Work out the finished part from the listing and answer in its coordinate system (mm). A direction names the side the tool comes from. Coordinates: 2 decimals unless noted, no trailing zeros. Order: outer loops, then holes, each group sorted by start corner. A loop starts at its lowest first (then second) coordinate and runs counter-clockwise, first axis right, second up. Notation, with made-up numbers: (23.5, 21.25) -> (68.5, 21.25) arc R30 cw to (68.5, 45.25) -> close; hole circle Ø8 at (10.5, -5.5). An arc over 180 degrees is marked (long way). Use one line per item in the form item = value.
from build123d import *

# Parameters (mm, degrees)
F1_DEPTH = 50


with BuildPart() as f1:
    # F0 (on Top) → F1 (new body)
    with BuildSketch(Plane.XY):
        with BuildLine():
            Line((-20.484694, -18.369378), (-21.890144, -14.507935))
            ThreePointArc((-21.890144, -14.507935), (-22.407219, -13.943648), (-23.171857, -13.910263))
            ThreePointArc((-23.171857, -13.910263), (-23.736145, -14.427337), (-23.76953, -15.191975))
            Line((-23.76953, -15.191975), (-22.364079, -19.053418))
            ThreePointArc((-22.364079, -19.053418), (-22.725701, -21.800208), (-25.183157, -23.079479))
            Line((-25.183157, -23.079479), (-58.007304, -23.079479))
            ThreePointArc((-58.007304, -23.079479), (-60.692462, -21.41736), (-60.402253, -18.272763))
            Line((-60.402253, -18.272763), (-39.547274, 9.372207))
            ThreePointArc((-39.547274, 9.372207), (-39.355248, 10.113094), (-39.743351, 10.772762))
            ThreePointArc((-39.743351, 10.772762), (-40.484238, 10.964788), (-41.143906, 10.576685))
            Line((-41.143906, 10.576685), (-61.998885, -17.068286))
            ThreePointArc((-61.998885, -17.068286), (-62.482568, -22.309281), (-58.007304, -25.079479))
            Line((-58.007304, -25.079479), (-25.183157, -25.079479))
            ThreePointArc((-25.183157, -25.079479), (-21.087397, -22.947361), (-20.484694, -18.369378))
        make_face()
    extrude(amount=F1_DEPTH)


solid = f1.part
(1) Section D-D on x = -37.5 is taken. Write down the section's boundary in (y, z), plus the area to 3 significant figures.
Data:
outline = (-25.08, 0) -> (-23.08, 0) -> (-23.08, 50) -> (-25.08, 50) -> close
area = 100 mm²
(2) Each of these flat-tipped pins is pushed along its axis until it touches: P1, Ø8, axis at y = 4.5, z = 30.5, coming from the +X side; P2, Ø8, axis at x = -56, z = 20.5, coming from the +Y side; P3, Ø1, axis at y = -15, z = 16, coming from the -X side. Where does it stop, or does it pass through?
Data:
P1 = -40.21
P2 = -3.81
P3 = -60.82
(3) Which of the six approach directions +Z, -Z, +X, -X, +Y, -Y give full straight-line access (tool end or side, diameter ignored) to faces 5 (the flat face through (-50.12, -4.64, 24.65)), 6 (the cylindrical face through (-21.126, -23.002, 24.65))?
Data:
face_5 = +Z, -Z
face_6 = +Z, -Z, +X
(4) Section C-C on z = 29 is taken. Write down the section's boundary in (x, y).
Data:
outline = (-62, -17.07) arc R5 ccw to (-58.01, -25.08) -> (-25.18, -25.08) arc R5 ccw to (-20.48, -18.37) -> (-21.89, -14.51) arc R1 ccw to (-23.17, -13.91) arc R1 ccw to (-23.77, -15.19) -> (-22.36, -19.05) arc R3 cw to (-25.18, -23.08) -> (-58.01, -23.08) arc R3 cw to (-60.4, -18.27) -> (-39.55, 9.37) arc R1 ccw to (-41.14, 10.58) -> close
(5) Straight lines are drawn through the part: line 1 along X through (y, z) = (-19, 7.5); line 2 along X through (y, z) = (-21.5, 29); line 3 along Y through (x, z) = (-32, 45). For each, find the intervals that lie inside material, in ascending order.
Data:
line_1 = -62.89 to -60.81, -22.38 to -20.3
line_2 = -62.8 to -60.65, -22.54 to -20.39
line_3 = -25.08 to -23.08
(6) The mould has two halves that part along X. Classify faces 1 (the flat face through (-51.425, -3.052, 24.65)), 2 (the flat face through (-23.077, -17.096, 24.65)), 3 (the flat face through (-51.2, -5.6, 0)), 4 (the cylindrical face through (-60.67, -21.46, 24.65)): released by +X, released by -X, zero draft, split by the parting line, or undercut.
Data:
face_1 = released by -X
face_2 = undercut
face_3 = zero draft
face_4 = undercut
(7) Section A-A on y = -20 is taken. Write down the section's boundary in (x, z).
Data:
outline = (-63.01, 0) -> (-61.01, 0) -> (-61.01, 50) -> (-63.01, 50) -> close; (-22.18, 0) -> (-20.18, 0) -> (-20.18, 50) -> (-22.18, 50) -> close
(8) Section B-B on x = -42 is taken. Write down the section's boundary in (y, z), plus the area to 3 significant figures.
Data:
outline = (-25.08, 0) -> (-23.08, 0) -> (-23.08, 50) -> (-25.08, 50) -> close; (6.12, 0) -> (9.44, 0) -> (9.44, 50) -> (6.12, 50) -> close
area = 266 mm²
